Verification items for the finished model (mm, model axes). A direction names the side the tool comes from. Coordinates: 2 decimals unless noted, no trailing zeros. Order: outer loops, then holes, each group sorted by start corner. A loop starts at its lowest first (then second) coordinate and runs counter-clockwise, first axis right, second up. Notation, with made-up numbers: M 71.5,66 L 116.5,66 A11 ccw 116.5,70 Z; hole C -39.75,-37.5 d3. An arc over 180 degrees is marked long. Return JSON: item names as keys, results as strings. Group by question number.
Q1. Section check A-A, the plane x = -5. Enter the section's corners in (y, z).
Q2. Section check C-C, the plane z = 12. Enter the section's corners in (x, y), then the cut area to 3 significant figures.
Q3. Access from +Z, -Z, +X, -X, +Y, -Y to the whole of each face (thin tool, end or side, straight path). Record for faces 5 (the face through (1, 25, 25)), 6 (the face through (-10, 63, 12)), 7 (the face through (-4.93, 60.6, 24.43)), 8 (the face through (-4, 60, 12)), 9 (the face through (1.5, 32, 12)).
Q4. Thickness scan on probe 1 along Z at (x, y) = (-5, 63.9); probe 2 along Z at (x, y) = (-5, 61.35); probe 3 along X at (y, z) = (25, 17). Record the ranges inside material, lowest first.
Q5. Mould release check, pull along Z, two halves, no side actions. Record for faces 1 (the face through (-7.385, 62.535, 7.001)), 2 (the face through (-9.43, 60.6, 12.68)), 3 (the face through (-4.93, 60.6, 0.57)), 4 (the face through (-6.34, 62.54, 20.86)): pulls with the +Z half, pulls with the -Z half, needs draft (parallel to the pull), parting line crosses it, or undercut.
Q6. Go/stop test with flat-tipped pins: pin 1 Ø7 at (x, z) = (7, 9) entering from +Y; pin 2 Ø2 at (y, z) = (16, 10) entering from +X; pin 3 Ø7.5 at (y, z) = (12, 7) entering from -X. Record where each tip stops, or that it passes through.
Q7. Section check B-B, the plane z = 18.75. Enter the section's corners in (x, y).
Q8. Section check D-D, the plane x = -1. Enter the section's corners in (y, z), then the cut area to 3 significant figures.
from build123d import *

# Parameters (mm, degrees)
F0_W     = 10
F0_H     = 5
F1_DEPTH = 25
F3_D     = 5
F4_R     = 2


# Not quite as in the source:
# - a feature names something its author has since deleted; it is built from what else it names


with BuildPart() as f1:
    # F0 (on Top) → F1 (new body)
    with BuildSketch(Plane.XY):
        Polygon((0, 60), (0, 0), (1.5, 0), (1.5, 65), (0, 65), align=None)
        with Locations((-5, 62.5)):
            Rectangle(F0_W, F0_H)
        Polygon((1.5, 0), (0, 0), (0, -15), (10, 0), align=None)
    extrude(amount=F1_DEPTH)

    # F3 (through all)
    with Locations(Plane.XZ.offset(-60)):
        with Locations((-5, 18.75), (-5, 6.25)):
            Hole(F3_D / 2)

    # F4
    f4_edges = [f1.edges().sort_by_distance(p)[0] for p in [
        (-10, 60, 12.5),
        (-5, 60, 25),
        (-5, 60, 0),
    ]]
    fillet(f4_edges, radius=F4_R)


solid = f1.part
Numbers:
{
 "1": {"outline": "M 60,2 A2 ccw 62,0 L 65,0 L 65,3.75 L 60,3.75 Z; M 60,8.75 L 65,8.75 L 65,16.25 L 60,16.25 Z; M 60,21.25 L 65,21.25 L 65,25 L 62,25 A2 ccw 60,23 Z"},
 "2": {"outline": "M -10,62 A2 ccw -8,60 L 0,60 L 0,-15 L 10,0 L 1.5,0 L 1.5,65 L -10,65 Z", "area": "222 mm2"},
 "3": {"face 5": "+Z, +X, -X, +Y, -Y", "face 6": "+Z, -Z, -X, +Y, -Y", "face 7": "+Z, -X, -Y", "face 8": "+Z, -Z, -X, -Y", "face 9": "+Z, -Z, +X, +Y"},
 "4": {"probe 1": "z = 0 to 3.75, 8.75 to 16.25, 21.25 to 25", "probe 2": "z = 0.11 to 3.75, 8.75 to 16.25, 21.25 to 24.89", "probe 3": "x = 0 to 1.5"},
 "5": {"face 1": "undercut", "face 2": "needs draft", "face 3": "pulls with the -Z half", "face 4": "undercut"},
 "6": {"pin 1": "stops at y = 0", "pin 2": "stops at x = 1.5", "pin 3": "stops at x = 0"},
 "7": {"outline": "M -10,62 A2 ccw -8,60 L -7.5,60 L -7.5,65 L -10,65 Z; M -2.5,60 L 0,60 L 0,-15 L 10,0 L 1.5,0 L 1.5,65 L -2.5,65 Z"},
 "8": {"outline": "M 60,2 A2 ccw 62,0 L 65,0 L 65,25 L 62,25 A2 ccw 60,23 Z", "area": "123 mm2"}
}
